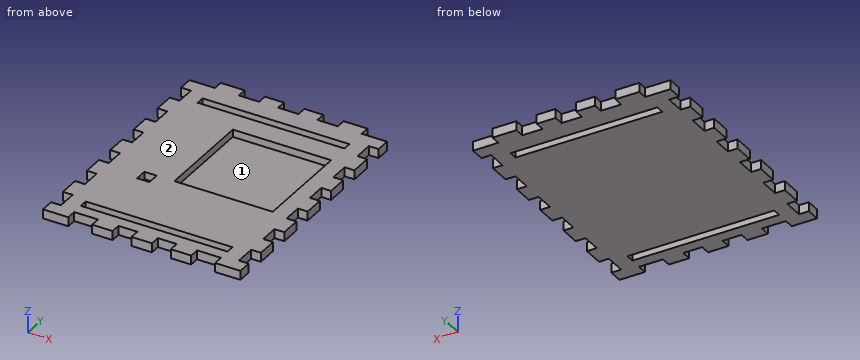
from build123d import *

# Parameters (mm, degrees)
MODEL_W             = 59.689998908
MODEL_H             = 3.386668819
MODEL_H_2           = 3.3866668
BOSS_EXTRUDE1_DEPTH = 3.7
SKETCH1_W           = 2.5
SKETCH1_H           = 2.5
SKETCH1_W_2         = 40
SKETCH1_H_2         = 40
CUT_EXTRUDE1_DEPTH  = 3


with BuildPart() as part:
    # Model → Boss-Extrude1 (new body)
    with BuildSketch(Plane.XY):
        Polygon((7.659321824, 131.185313162), (11.645711781, 131.185313467), (11.645711781, 123.120135193), (7.659323163, 123.120135799), (7.659323163, 114.794580784), (11.645711704, 114.794580995), (11.645711704, 106.729402721), (7.659323085, 106.729402721), (7.659322496, 101.163927511), (17.960431856, 101.163927511), (17.960431856, 105.185592023), (27.661820742, 105.185592023), (27.661820742, 101.163927511), (35.952098518, 101.163927511), (35.952098518, 105.185592023), (43.642655148, 105.185592023), (43.642655148, 101.163927511), (51.968212855, 101.163927511), (51.968212855, 105.185592023), (59.658766793, 105.185592023), (59.658766793, 101.163927511), (67.949044569, 101.163927511), (67.949044569, 105.185592023), (77.650433456, 105.185592023), (77.650433456, 101.163927511), (87.951545673, 101.163927511), (87.951545673, 106.78652537), (83.965155709, 106.78652537), (83.965155709, 115.20447842), (87.951545673, 115.204478756), (87.951545673, 123.494756532), (83.965155708, 123.494756532), (83.965155708, 131.185313162), (87.951545168, 131.185313162), (87.951545168, 139.475590938), (83.965156213, 139.475590938), (83.965156213, 147.166147568), (87.951545168, 147.166147568), (87.951545168, 155.456425344), (83.965156213, 155.456425344), (83.965156213, 163.182259213), (87.951545168, 163.182259213), (87.951545168, 171.472536989), (83.965156213, 171.472536989), (83.965156213, 179.163092274), (87.951545169, 179.163092274), (87.951545169, 187.851347209), (84.066213746, 187.851347204), (83.965155204, 195.685953684), (87.951545169, 195.685953684), (87.951544665, 201.458647414), (77.650433455, 201.458647414), (77.650433455, 205.445036033), (67.949044569, 205.445036033), (67.949044569, 201.458647414), (59.658766793, 201.458647414), (59.658766793, 205.445036033), (51.968212854, 205.445036033), (51.968212854, 201.458647414), (43.642655148, 201.458647414), (43.642655148, 205.445036033), (35.952098517, 205.445036033), (35.952098517, 201.458647414), (27.661820742, 201.458647414), (27.661820742, 205.445036033), (17.960431855, 205.445036033), (17.960431855, 201.458647414), (7.659323162, 201.458647414), (7.659321865, 195.685953684), (11.645710483, 195.685953684), (11.645711788, 187.863269672), (7.65932317, 187.863269672), (7.65932317, 179.537714657), (11.645711788, 179.537715263), (11.645711788, 171.472536989), (7.659321824, 171.472536989), (7.659321824, 163.182259214), (11.645711789, 163.182259214), (11.645711789, 155.456425344), (7.659321824, 155.456425344), (7.659321824, 147.166147568), (11.645711789, 147.166147568), (11.645711789, 139.475590938), (7.659321824, 139.475590938), align=None)
        with Locations((47.664322352, 111.627811013)):
            Rectangle(MODEL_W, MODEL_H, mode=Mode.SUBTRACT)
        with Locations((47.664322352, 191.629758602)):
            Rectangle(MODEL_W, MODEL_H_2, mode=Mode.SUBTRACT)
    extrude(amount=BOSS_EXTRUDE1_DEPTH)

    # Sketch1 → Cut-Extrude1 (cut)
    with BuildSketch(Plane.XY.offset(3.7)):
        with Locations((26.569322898, 137.071145422)):
            Rectangle(SKETCH1_W, SKETCH1_H)
        Polygon((27.819322898, 138.321145422), (27.819322898, 135.821145422), (30.319322898, 135.821145422), (30.319322898, 140.821145422), (25.319322898, 140.821145422), (25.319322898, 138.321145422), align=None)
        with Locations((57.509321806, 160.821145422)):
            Rectangle(SKETCH1_W_2, SKETCH1_H_2)
    extrude(amount=-CUT_EXTRUDE1_DEPTH, mode=Mode.SUBTRACT)


solid = part.part
Can you work these out from the model? Positions are in its coordinate system, mm. Face numbers are marked on the shaded views. Coordinates: 2 decimals unless noted, no trailing zeros. Write each loop counter-clockwise with the first axis right and the second up, starting at its lowest first coordinate (ties: lowest second). Pieces come first, ordered by that corner, then holes. Notation, with made-up numbers: (38.25, 76.5) -> (50.25, 76.5) arc R23 cw to (50.25, 85.5) -> close; hole circle Ø2 at (-8.5, 8). An arc over 180 degrees is marked (long way). Answer as CSV lines item,"result".
1) If we section it at B-B on x = 32: Please give me the cut outline in (y, z).
Check result:
outline,"(101.16, 0) -> (109.93, 0) -> (109.93, 3.7) -> (101.16, 3.7) -> close; (113.32, 0) -> (189.94, 0) -> (189.94, 3.7) -> (113.32, 3.7) -> close; (193.32, 0) -> (201.46, 0) -> (201.46, 3.7) -> (193.32, 3.7) -> close"
2) If we section it at D-D on y = 178: Please give me the cut outline in (x, z), then the cut area to 3 significant figures.
Check result:
outline,"(11.65, 0) -> (83.97, 0) -> (83.97, 3.7) -> (77.51, 3.7) -> (77.51, 0.7) -> (37.51, 0.7) -> (37.51, 3.7) -> (11.65, 3.7) -> close"
area,"148 mm²"
3) If I drill on line 1 (Y direction, x = 27, z = 1.9); line 2 (Y direction, x = 20.5, z = 3.1); line 3 (Y direction, x = 46.5, z = 3.05), over which ranges is the centre line in solid material (lowest first)? Write a range as from..to.
Check result:
line 1,"105.19..109.93, 113.32..135.82, 140.82..189.94, 193.32..205.45"
line 2,"105.19..109.93, 113.32..189.94, 193.32..205.45"
line 3,"101.16..109.93, 113.32..140.82, 180.82..189.94, 193.32..201.46"
4) Will these pins go through, and if not, where does the flat tip stop? P1, Ø1.1, axis at y = 159.5, z = 2, coming from the +X side; P2, Ø1.8, axis at x = 46.5, z = 2.5, coming from the +Y side; P3, Ø1.7, axis at y = 192.5, z = 1.5, coming from the -X side.
Check result:
P1,"x = 83.97"
P2,"y = 201.46"
P3,"x = 11.65"
5) If we section it at A-A on x = 20.5: Please give me the cut outline in (y, z), then the cut area to 3 significant figures.
Check result:
outline,"(105.19, 0) -> (109.93, 0) -> (109.93, 3.7) -> (105.19, 3.7) -> close; (113.32, 0) -> (189.94, 0) -> (189.94, 3.7) -> (113.32, 3.7) -> close; (193.32, 0) -> (205.45, 0) -> (205.45, 3.7) -> (193.32, 3.7) -> close"
area,"346 mm²"
6) If we section it at C-C on z = 2.55: Count the separate pieces of the cut face and the enclosed holes in it, then the cut area to 3 significant figures.
Check result:
separate pieces,"1"
enclosed holes,"4"
area,"5,650 mm²"
7) If we mould it in two halves opening along Y, with no side actions, what happens to the marked faces 1 and 2? For each: +Y half, -Y half, draft (parallel to the pull), parting line (faces both ways), or undercut.
Check result:
face 1,"undercut"
face 2,"draft"
